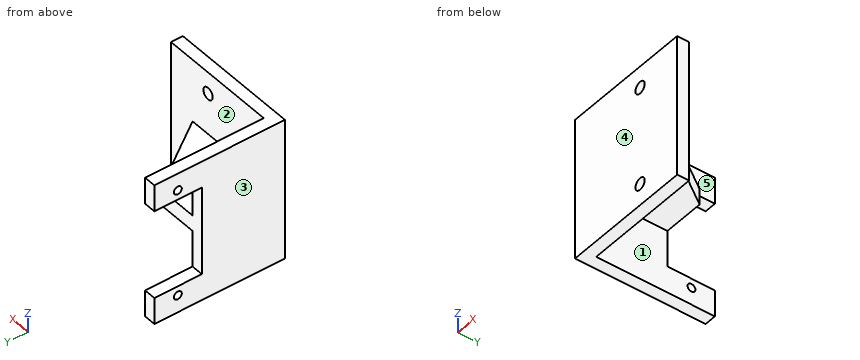
from build123d import *

# Parameters (mm, degrees)
EXTRUDE_THIN1_DEPTH = 18
SKETCH2_W           = 22.5
SKETCH2_H           = 12
CUT_EXTRUDE1_DEPTH  = 4
SKETCH3_R           = 1
CUT_EXTRUDE2_DEPTH  = 4
SKETCH6_W           = 23
SKETCH6_H           = 4
BOSS_EXTRUDE1_DEPTH = 18
CUT_EXTRUDE3_DEPTH  = 21
SKETCH8_R           = 1.5
CUT_EXTRUDE4_DEPTH  = 4


with BuildPart() as part:
    # Sketch1 → Extrude-Thin1 (new body, symmetric)
    with BuildSketch(Plane.XY):
        Polygon((30, 0), (0, 0), (0, 30), (-3, 30), (-3, -3), (30, -3), align=None)
    extrude(amount=EXTRUDE_THIN1_DEPTH, both=True)

    # Sketch2 → Cut-Extrude1 (cut, through all)
    with BuildSketch(Plane(origin=(0, 0, 0), x_dir=(0, 0, -1), z_dir=(1, 0, 0))):
        with Locations((0, 24)):
            Rectangle(SKETCH2_W, SKETCH2_H)
    extrude(amount=-CUT_EXTRUDE1_DEPTH, mode=Mode.SUBTRACT)

    # Sketch3 → Cut-Extrude2 (cut, through all)
    with BuildSketch(Plane(origin=(0, 0, 0), x_dir=(0, 0, -1), z_dir=(1, 0, 0))):
        with Locations((13.625, 24.069423531)):
            Circle(SKETCH3_R)
        with Locations((-13.625, 24.069423531)):
            Circle(SKETCH3_R)
    extrude(amount=-CUT_EXTRUDE2_DEPTH, mode=Mode.SUBTRACT)

    # Sketch6 → Boss-Extrude1 (add)
    with BuildSketch(Plane(origin=(0, 0, 0), x_dir=(1, 0, 0), z_dir=(0, 1, 0))):
        with Locations((11.5, 0)):
            Rectangle(SKETCH6_W, SKETCH6_H)
    extrude(amount=BOSS_EXTRUDE1_DEPTH)

    # Sketch7 → Cut-Extrude3 (cut, through all)
    with BuildSketch(Plane(origin=(0, 0, -2), x_dir=(-1, 0, 0), z_dir=(0, 0, -1))):
        Polygon((-10.399594351, 18), (-23, 18), (-23, 0), align=None)
    extrude(amount=-CUT_EXTRUDE3_DEPTH, mode=Mode.SUBTRACT)

    # Sketch8 → Cut-Extrude4 (cut, through all)
    with BuildSketch(Plane(origin=(0, 0, 0), x_dir=(1, 0, 0), z_dir=(0, 1, 0))):
        with Locations((18, 12.5)):
            Circle(SKETCH8_R)
        with Locations((18, -12.5)):
            Circle(SKETCH8_R)
    extrude(amount=-CUT_EXTRUDE4_DEPTH, mode=Mode.SUBTRACT)


solid = part.part
Can you work these out from the model? Positions are in its coordinate system, mm. Face numbers are marked on the shaded views. A direction names the side the tool comes from. Coordinates: 2 decimals unless noted, no trailing zeros. Order: outer loops, then holes, each group sorted by start corner. A loop starts at its lowest first (then second) coordinate and runs counter-clockwise, first axis right, second up. Notation, with made-up numbers: M 81,-18.5 L 124,-18.5 A24 ccw 124,1.5 Z; hole C -37,47.25 d11. An arc over 180 degrees is marked long. Write item = value, one per line.
(1) Suppose I cut it at A-A on x = 7. Please give me the cut outline in (y, z).
Results are:
outline = M -3,-18 L 0,-18 L 0,-2 L 18,-2 L 18,2 L 0,2 L 0,18 L -3,18 Z
(2) For pin 1 Ø5 at (y, z) = (19, -8) entering from +X; pin 2 Ø4 at (x, z) = (18, -12.5) entering from +Y; pin 3 Ø15 at (x, z) = (15, -5.5) entering from +Y, each with a flat end and sliding along its axis, tell me the tip position at first contact or that it passes through.
Results are:
pin_1 = 0
pin_2 = 0
pin_3 = 18
(3) Suppose I cut it at D-D on z = -3.5. Please give me the cut outline in (x, y), plus the area to 3 significant figures.
Results are:
outline = M -3,-3 L 30,-3 L 30,0 L 0,0 L 0,18 L -3,18 Z
area = 153 mm2
(4) For the marked faces 1, 2, 3, 4 and 5, which set-ups out of +Z, -Z, +X, -X, +Y, -Y let a thin tool reach every point of the face, with its end or its side?
Results are:
face_1 = -Z, +X, +Y
face_2 = +X, +Y
face_3 = +Z, -Z, -X, +Y, -Y
face_4 = +Z, -Z, +X, -X, -Y
face_5 = +Z, +X, +Y
(5) Suppose I cut it at B-B on x = 18. Please give me the cut outline in (y, z), plus the area to 3 significant figures.
Results are:
outline = M -3,-18 L 0,-18 L 0,-14 L -3,-14 Z; M -3,-11 L 0,-11 L 0,-2 L 7.14,-2 L 7.14,2 L 0,2 L 0,11 L -3,11 Z; M -3,14 L 0,14 L 0,18 L -3,18 Z
area = 119 mm2
(6) Suppose I cut it at C-C on y = 8.5. Please give me the cut outline in (x, z).
Results are:
outline = M -3,-18 L 0,-18 L 0,-2 L 17.05,-2 L 17.05,2 L 0,2 L 0,18 L -3,18 Z
(7) I need wall thicknesses on line 1 along X through (y, z) = (-0.8, 12.5); line 2 along Z through (x, y) = (18, -1); line 3 along X through (y, z) = (20, -14.5). Which ranges of each line are inside material? Lowest first, please. Write a range as [from, to].
Results are:
line_1 = [-3, 16.5], [19.5, 30]
line_2 = [-18, -14], [-11, 11], [14, 18]
line_3 = [-3, 0]
